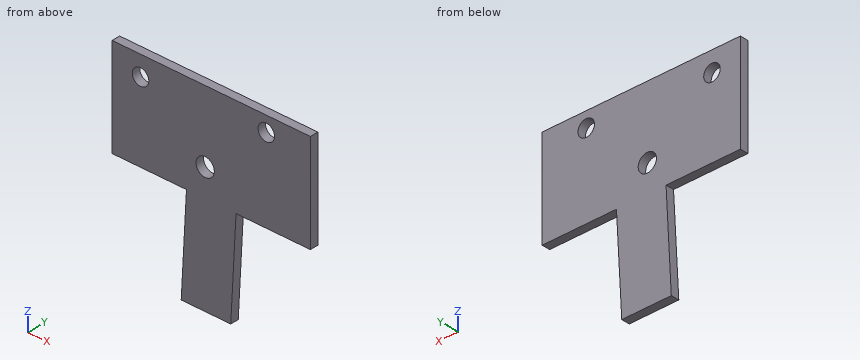
```python
from build123d import *

# Parameters (mm, degrees)
F1_DEPTH = 12.7
F2_R     = 12.7
F2_R_2   = 14.065671
F3_DEPTH = 61.214


with BuildPart() as f1:
    # F0 (on Front) → F1 (new body)
    with BuildSketch(Plane.XZ):
        Polygon((-77.600956, 42.763185), (36.699044, 42.763185), (28.587316, -109.420782), (104.787316, -109.420782), (112.899044, 42.763185), (227.199044, 42.763185), (227.199044, 195.163185), (-77.600956, 195.163185), align=None)
    extrude(amount=F1_DEPTH)

    # F2 (on face) → F3 (cut)
    with BuildSketch(Plane.XZ.offset(12.7)):
        with Locations((-33.92983, 164.380682)):
            Circle(F2_R)
        with Locations((65.435274, 85.294179)):
            Circle(F2_R_2)
        with Locations((159.39275, 171.816179)):
            Circle(F2_R)
    extrude(amount=-F3_DEPTH, mode=Mode.SUBTRACT)


solid = f1.part
```
Design review of the part built by this model. Coordinates are the model's own, in mm. Round coordinates to 2 decimals unless told otherwise and drop trailing zeros. Write each loop counter-clockwise with the first axis right and the second up, starting at its lowest first coordinate (ties: lowest second). Pieces come first, ordered by that corner, then holes. Notation, with made-up numbers: (79.5, -7.5) -> (109.5, -7.5) arc R19 ccw to (109.5, 6.5) -> close; hole circle Ø2 at (30, 76.5). An arc over 180 degrees is marked (long way). Answer in a Markdown table with one row per item.
Q1. Clearance check with flat-ended pins moving along their axes: pin 1 Ø1 at (y, z) = (-5.5, 15.5) entering from +X; pin 2 Ø1.5 at (y, z) = (-7.5, -12.5) entering from +X; pin 3 Ø6.5 at (x, y) = (160, -8) entering from -Z. State where each tip first meets the part, or that it passes through.
The answers:
| item | result |
|---|---|
| pin 1 | x = 111.47 |
| pin 2 | x = 109.99 |
| pin 3 | z = 42.76 |
Q2. To check wall thickness, follow L1, parallel to Z at x = 176.5, y = -5.5; L2, parallel to Z at x = 160, y = -1.75; L3, parallel to Z at x = -26.5, y = -7.5. State the ranges of each line that lie inside material, in increasing order. Write a range as [from, to].
The answers:
| item | result |
|---|---|
| L1 | [42.76, 195.16] |
| L2 | [42.76, 159.13], [184.5, 195.16] |
| L3 | [42.76, 154.08], [174.68, 195.16] |
Q3. Take a section at B-B, the plane z = 89. State the section outline as (x, y) points, then the cut area to 3 significant figures.
The answers:
| item | result |
|---|---|
| outline | (-77.6, -12.7) -> (51.87, -12.7) -> (51.87, 0) -> (-77.6, 0) -> close; (79, -12.7) -> (227.2, -12.7) -> (227.2, 0) -> (79, 0) -> close |
| area | 3,530 mm² |
Q4. Take a section at A-A, the plane x = 70. State the section outline as (y, z) points, then the cut area to 3 significant figures.
The answers:
| item | result |
|---|---|
| outline | (-12.7, -109.42) -> (0, -109.42) -> (0, 71.99) -> (-12.7, 71.99) -> close; (-12.7, 98.6) -> (0, 98.6) -> (0, 195.16) -> (-12.7, 195.16) -> close |
| area | 3,530 mm² |
Q5. Take a section at C-C, the plane y = -7.5. State the section outline as (x, z) points.
The answers:
| item | result |
|---|---|
| outline | (-77.6, 42.76) -> (36.7, 42.76) -> (28.59, -109.42) -> (104.79, -109.42) -> (112.9, 42.76) -> (227.2, 42.76) -> (227.2, 195.16) -> (-77.6, 195.16) -> close; hole circle Ø25.4 at (-33.93, 164.38); hole circle Ø28.13 at (65.44, 85.29); hole circle Ø25.4 at (159.39, 171.82) |
Q6. Take a section at D-D, the plane x = -59. State the section outline as (y, z) points, then the cut area to 3 significant figures.
The answers:
| item | result |
|---|---|
| outline | (-12.7, 42.76) -> (0, 42.76) -> (0, 195.16) -> (-12.7, 195.16) -> close |
| area | 1,940 mm² |
